Design review of the part built by this model. Coordinates are the model's own, in mm. Face numbers are marked on the shaded views. Give positions to 0.01 mm unless a question says otherwise; leave off trailing zeros. Loops run counter-clockwise (first coordinate to the right, second up) from the corner with the lowest first, then second, coordinate; pieces in that order, holes last. Notation, with made-up numbers: (29, -9) -> (70, -9) arc R20 ccw to (70, 22) -> close; hole circle Ø7 at (59.25, 9). An arc over 180 degrees is marked (long way). Answer in a Markdown table with one row per item. Add a question column.
(1) Consider section C-C on x = -18. Write out the cut boundary in (y, z).
(2) For line 1 (X direction, y = 0, z = -0.9); line 2 (X direction, y = 0, z = -2.15); line 3 (Y direction, x = 0, z = -10.25), list the stretches that pass through material, from the lowest coordinate up.
(3) For pin 1 (4 mm diameter, centred on x = 18.415, y = 0, fed in from -Z); pin 2 (6 mm diameter, centred on y = -23, z = -6, fed in from -X); pin 3 (8 mm diameter, centred on y = 25, z = -15, fed in from +X); pin 4 (4 mm diameter, centred on x = -5.5, z = -15.5, fed in from -Y), all flat-tipped, find the tip position at first contact; note any pin that passes through.
(4) Draft analysis for pull direction Y (two halves, no side actions). For the marked faces 1, 2 and 3, state which applies: +Y half, -Y half, draft (parallel to the pull), parting line (faces both ways), or undercut.
(5) Consider section D-D on y = 25.5. Write out the cut boundary in (x, z), then the cut area to 3 significant figures.
(6) Consider section B-B on y = 0. Count the separate pieces of the cut face and the enclosed holes in it, then the cut area to 3 significant figures.
from build123d import *

# Parameters (mm, degrees)
F2_R     = 3.2385
F3_DEPTH = 19.051
F4_W     = 1.6002
F4_H     = 1.6002
F6_W     = 1.6002
F6_H     = 1.6002
F8_SIZE  = 0.254


with BuildPart() as f1:
    # F0 (on Front) → F1 (revolve)
    with BuildSketch(Plane.XZ):
        Polygon((34, 0), (0, 0), (0, -19.05), (19.05, -19.05), (19.05, -17.4752), (22.225, -17.4752), (22.225, -19.05), (29, -19.05), (29, -1.6002), (34, -1.6002), align=None)
    revolve(axis=Axis((0, 0, -7.0298854262), (0, 0, -1)))

    # F2 (on face) → F3 (cut, through all)
    with BuildSketch(Plane(origin=(0, 0, -19.05), x_dir=(1, 0, 0), z_dir=(0, 0, -1))):
        Circle(F2_R)
        with Locations((18.415, 0)):
            Circle(F2_R)
    extrude(amount=-F3_DEPTH, mode=Mode.SUBTRACT)

    # F4 (on Front) → F5 (revolve, cut)
    with BuildSketch(Plane.XZ):
        with Locations((4.0386, -2.4003)):
            Rectangle(F4_W, F4_H)
    revolve(axis=Axis((0, 0, -2.3049995583), (0, 0, -1)), mode=Mode.SUBTRACT)

    # F6 (on Front) → F7 (revolve, cut)
    with BuildSketch(Plane.XZ):
        with Locations((22.4536, -2.4003)):
            Rectangle(F6_W, F6_H)
    revolve(axis=Axis((18.415, 0, -9.4374260038), (0, 0, -1)), mode=Mode.SUBTRACT)

    # F8
    f8_edges = [f1.edges().sort_by_distance(p)[0] for p in [
        (-3.2385, 0, 0),
        (15.1765, 0, 0),
    ]]
    chamfer(f8_edges, length=F8_SIZE)


solid = f1.part
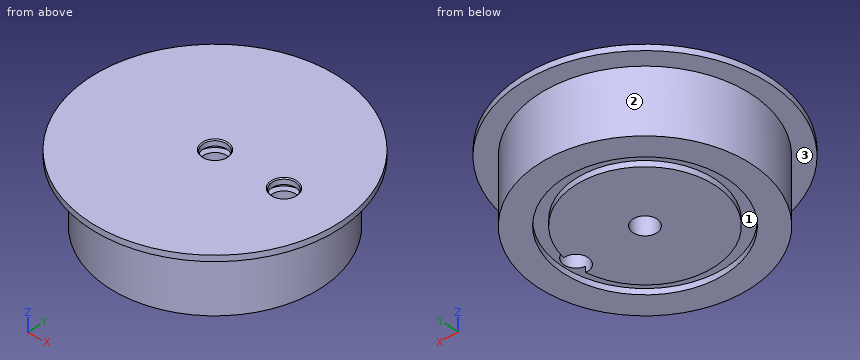
Values follow:
| question | item | result |
|---|---|---|
| 1 | outline | (-28.84, -1.6) -> (-22.74, -1.6) -> (-22.74, -19.05) -> (-13.04, -19.05) -> (-13.04, -17.48) -> (-6.24, -17.48) -> (-6.24, -19.05) -> (6.24, -19.05) -> (6.24, -17.48) -> (13.04, -17.48) -> (13.04, -19.05) -> (22.74, -19.05) -> (22.74, -1.6) -> (28.84, -1.6) -> (28.84, 0) -> (-28.84, 0) -> close |
| 2 | line 1 | -34 to -3.24, 3.24 to 15.18, 21.65 to 34 |
| 2 | line 2 | -29 to -4.84, 4.84 to 13.58, 23.25 to 29 |
| 2 | line 3 | -29 to -3.24, 3.24 to 29 |
| 3 | pin 1 | through |
| 3 | pin 2 | x = -21 |
| 3 | pin 3 | x = 20 |
| 3 | pin 4 | y = -28.79 |
| 4 | face 1 | undercut |
| 4 | face 2 | parting line |
| 4 | face 3 | draft |
| 5 | outline | (-22.49, -1.6) -> (-13.81, -1.6) -> (-13.81, -19.05) -> (13.81, -19.05) -> (13.81, -1.6) -> (22.49, -1.6) -> (22.49, 0) -> (-22.49, 0) -> close |
| 5 | area | 554 mm2 |
| 6 | separate pieces | 3 |
| 6 | enclosed holes | 0 |
| 6 | area | 858 mm2 |
